from build123d import *

# Parameters (mm, degrees)
SKETCH1_W           = 463.88
SKETCH1_H           = 60
BOSS_EXTRUDE1_DEPTH = 3.175
SKETCH7_R           = 2.5
CUT_EXTRUDE5_DEPTH  = 448.729854963
SKETCH2_R           = 1.25
SKETCH2_R_2         = 1.5
SKETCH2_W           = 103
SKETCH2_H           = 37
CUT_EXTRUDE1_DEPTH  = 448.729854963
SKETCH3_W           = 158.75
SKETCH3_H           = 44.7
CUT_EXTRUDE2_DEPTH  = 448.729854963
SKETCH4_R           = 18
SKETCH4_W           = 38.5
SKETCH4_H           = 30.5
CUT_EXTRUDE3_DEPTH  = 448.729854963
SKETCH5_W           = 31.25
SKETCH5_H           = 6.35
SKETCH5_W_2         = 20
SKETCH5_W_3         = 74.25
SKETCH5_W_4         = 59.87
BOSS_EXTRUDE2_DEPTH = 3.175
SKETCH6_R           = 1.5
CUT_EXTRUDE4_DEPTH  = 449.624949735
SKETCH8_R           = 1
CUT_EXTRUDE7_DEPTH  = 449.624949735
CHAMFER2_SIZE       = 0.8


with BuildPart() as part:
    # Sketch1 → Boss-Extrude1 (new body)
    with BuildSketch(Plane(origin=(0, 0, 0), x_dir=(-1, 0, 0), z_dir=(0, 0, -1))):
        with Locations((-211.74, 30)):
            Rectangle(SKETCH1_W, SKETCH1_H)
    extrude(amount=BOSS_EXTRUDE1_DEPTH)

    # Sketch7 → Cut-Extrude5 (cut, through all)
    with BuildSketch(Plane(origin=(0, 0, -3.175), x_dir=(-1, 0, 0), z_dir=(0, 0, -1))):
        with Locations((-433.68, 50)):
            Circle(SKETCH7_R)
        with Locations((-433.68, 10)):
            Circle(SKETCH7_R)
        with Locations((10.2, 10)):
            Circle(SKETCH7_R)
        with Locations((10.2, 50)):
            Circle(SKETCH7_R)
    extrude(amount=-CUT_EXTRUDE5_DEPTH, mode=Mode.SUBTRACT)

    # Sketch2 → Cut-Extrude1 (cut, through all)
    with BuildSketch(Plane(origin=(0, 0, -3.175), x_dir=(-1, 0, 0), z_dir=(0, 0, -1))):
        with Locations((-106.378679656, 39)):
            Circle(SKETCH2_R)
        with Locations((-222.5, 49)):
            Circle(SKETCH2_R_2)
        with Locations((-222.5, 29)):
            Circle(SKETCH2_R_2)
        with Locations((-166, 37.5)):
            Rectangle(SKETCH2_W, SKETCH2_H)
        with BuildLine():
            Line((-217.5, 13), (-217.5, 18.9))
            Line((-217.5, 18.9), (-214.5, 18.9))
            Line((-214.5, 18.9), (-214.5, 13))
            ThreePointArc((-214.5, 13), (-216, 11.5), (-217.5, 13))
        make_face()
    extrude(amount=-CUT_EXTRUDE1_DEPTH, mode=Mode.SUBTRACT)

    # Sketch3 → Cut-Extrude2 (cut, through all)
    with BuildSketch(Plane(origin=(0, 0, -3.175), x_dir=(-1, 0, 0), z_dir=(0, 0, -1))):
        with Locations((-336.745, 26.05)):
            Rectangle(SKETCH3_W, SKETCH3_H)
    extrude(amount=-CUT_EXTRUDE2_DEPTH, mode=Mode.SUBTRACT)

    # Sketch4 → Cut-Extrude3 (cut, through all)
    with BuildSketch(Plane(origin=(0, 0, -3.175), x_dir=(-1, 0, 0), z_dir=(0, 0, -1))):
        with Locations((-60.25, 20.25)):
            Circle(SKETCH4_R)
        with BuildLine():
            Line((-77.75, 4.25), (-77.75, 5.25))
            ThreePointArc((-77.75, 5.25), (-76.25, 6.75), (-74.75, 5.25))
            Line((-74.75, 5.25), (-74.75, 4.25))
            ThreePointArc((-74.75, 4.25), (-76.25, 2.75), (-77.75, 4.25))
        make_face()
        with BuildLine():
            Line((-77.75, 36.25), (-77.75, 37.25))
            ThreePointArc((-77.75, 37.25), (-76.25, 38.75), (-74.75, 37.25))
            Line((-74.75, 37.25), (-74.75, 36.25))
            ThreePointArc((-74.75, 36.25), (-76.25, 34.75), (-77.75, 36.25))
        make_face()
        with BuildLine():
            Line((-16.7, 3.5), (-16.7, 4.5))
            ThreePointArc((-16.7, 4.5), (-15.2, 6), (-13.7, 4.5))
            Line((-13.7, 4.5), (-13.7, 3.5))
            ThreePointArc((-13.7, 3.5), (-15.2, 2), (-16.7, 3.5))
        make_face()
        with BuildLine():
            Line((-5.9, 4.5), (-5.9, 5.5))
            ThreePointArc((-5.9, 5.5), (-4.4, 7), (-2.9, 5.5))
            Line((-2.9, 5.5), (-2.9, 4.5))
            ThreePointArc((-2.9, 4.5), (-4.4, 3), (-5.9, 4.5))
        make_face()
        with Locations((-20.75, 23.75)):
            Rectangle(SKETCH4_W, SKETCH4_H)
    extrude(amount=-CUT_EXTRUDE3_DEPTH, mode=Mode.SUBTRACT)

    # Sketch5 → Boss-Extrude2 (add)
    with BuildSketch(Plane(origin=(0, 0, -3.175), x_dir=(-1, 0, 0), z_dir=(0, 0, -1))):
        with Locations((-65.875, -3.175)):
            Rectangle(SKETCH5_W, SKETCH5_H)
        with Locations((-9.8, -3.175)):
            Rectangle(SKETCH5_W_2, SKETCH5_H)
        with Locations((-87.375, 63.175)):
            Rectangle(SKETCH5_W_3, SKETCH5_H)
        with Locations((-237.435, 63.175)):
            Rectangle(SKETCH5_W_4, SKETCH5_H)
        with Locations((-237.435, -3.175)):
            Rectangle(SKETCH5_W_4, SKETCH5_H)
        with Locations((-413.68, 63.175)):
            Rectangle(SKETCH5_W_2, SKETCH5_H)
        with Locations((-413.68, -3.175)):
            Rectangle(SKETCH5_W_2, SKETCH5_H)
    extrude(amount=-BOSS_EXTRUDE2_DEPTH)

    # Sketch6 → Cut-Extrude4 (cut, through all)
    with BuildSketch(Plane(origin=(0, 0, -3.175), x_dir=(-1, 0, 0), z_dir=(0, 0, -1))):
        with Locations((-247.37, 50)):
            Circle(SKETCH6_R)
        with Locations((-233.5, 10)):
            Circle(SKETCH6_R)
    extrude(amount=-CUT_EXTRUDE4_DEPTH, mode=Mode.SUBTRACT)

    # Sketch8 → Cut-Extrude7 (cut, through all)
    with BuildSketch(Plane(origin=(0, 0, -3.175), x_dir=(-1, 0, 0), z_dir=(0, 0, -1))):
        with Locations((-415.412893219, 47.692893219)):
            Circle(SKETCH8_R)
        with Locations((-258.077106781, 47.692893219)):
            Circle(SKETCH8_R)
        with Locations((-258.077106781, 4.407106781)):
            Circle(SKETCH8_R)
        with Locations((-415.412893219, 4.407106781)):
            Circle(SKETCH8_R)
        with Locations((-216.792893219, 55.292893219)):
            Circle(SKETCH8_R)
        with Locations((-115.207106781, 55.292893219)):
            Circle(SKETCH8_R)
        with Locations((-115.207106781, 19.707106781)):
            Circle(SKETCH8_R)
        with Locations((-424.387106781, 60.707106781)):
            Circle(SKETCH8_R)
        with Locations((-402.972893219, 60.707106781)):
            Circle(SKETCH8_R)
        with Locations((-268.077106781, 60.707106781)):
            Circle(SKETCH8_R)
        with Locations((-206.792893219, 60.707106781)):
            Circle(SKETCH8_R)
        with Locations((-125.207106781, 60.707106781)):
            Circle(SKETCH8_R)
        with Locations((-49.542893219, 60.707106781)):
            Circle(SKETCH8_R)
        with Locations((0.907106781, -0.707106781)):
            Circle(SKETCH8_R)
        with Locations((-20.507106781, -0.707106781)):
            Circle(SKETCH8_R)
        with Locations((-49.542893219, -0.707106781)):
            Circle(SKETCH8_R)
        with Locations((-82.207106781, -0.707106781)):
            Circle(SKETCH8_R)
        with Locations((-206.792893219, -0.707106781)):
            Circle(SKETCH8_R)
        with Locations((-268.077106781, -0.707106781)):
            Circle(SKETCH8_R)
        with Locations((-402.972893219, -0.707106781)):
            Circle(SKETCH8_R)
        with Locations((-424.387106781, -0.707106781)):
            Circle(SKETCH8_R)
        with Locations((-39.292893219, 38.292893219)):
            Circle(SKETCH8_R)
        with Locations((-2.207106781, 38.292893219)):
            Circle(SKETCH8_R)
        with Locations((-39.292893219, 9.207106781)):
            Circle(SKETCH8_R)
        with Locations((-2.207106781, 9.207106781)):
            Circle(SKETCH8_R)
    extrude(amount=-CUT_EXTRUDE7_DEPTH, mode=Mode.SUBTRACT)

    # Chamfer2
    chamfer2_edges = [part.edges().sort_by_distance(p)[0] for p in [
        (81.5, -6.35, -1.5875),
        (50.25, -6.35, -1.5875),
        (19.8, -6.35, -1.5875),
        (-0.2, -6.35, -1.5875),
        (124.5, 66.35, -1.5875),
        (50.25, 66.35, -1.5875),
        (267.37, 66.35, -1.5875),
        (207.5, 66.35, -1.5875),
        (267.37, -6.35, -1.5875),
        (207.5, -6.35, -1.5875),
        (423.68, -6.35, -1.5875),
        (403.68, -6.35, -1.5875),
        (403.68, 66.35, -1.5875),
        (423.68, 66.35, -1.5875),
    ]]
    chamfer(chamfer2_edges, length=CHAMFER2_SIZE)


solid = part.part
The listing builds one solid part. Answer for the finished solid, in the listing's coordinates (mm). Give positions to 0.01 mm unless a question says otherwise; leave off trailing zeros. Loops run counter-clockwise (first coordinate to the right, second up) from the corner with the lowest first, then second, coordinate; pieces in that order, holes last.
Item 1: Each of these flat-tipped pins is pushed along its axis until it touches: pin 1 Ø1 at (y, z) = (63, -2) entering from -X; pin 2 Ø2 at (x, y) = (106.38, 39) entering from +Z; pin 3 Ø1 at (x, z) = (430.5, -2.5) entering from -Y. Where does it stop, or does it pass through?
Derived:
pin 1: stops at x = 50.25
pin 2: passes through
pin 3: stops at y = 0
Item 2: A cutting plane is placed at A-A (x = 293.5). Give the vertices of the cut face in (y, z) (3 decimals), then the cut area to 3 significant figures.
Derived:
outline: (0, -3.175) - (3.7, -3.175) - (3.7, 0) - (0, 0) - close; (48.4, -3.175) - (60, -3.175) - (60, 0) - (48.4, 0) - close
area: 48.6 mm2
Item 3: Find the intervals of material crossed by line 1 along X through (y, z) = (-3, -0.7); line 2 along Y through (x, z) = (20, -2.9); line 3 along Y through (x, z) = (368.5, -0.4), in increasing order.
Derived:
line 1: x = -0.2 to 19.8, 50.25 to 81.5, 207.5 to 267.37, 403.68 to 423.68
line 2: y = 0.15 to 8.5, 39 to 60
line 3: y = 0 to 3.7, 48.4 to 60
Item 4: A cutting plane is placed at B-B (z = -1.35). Give the number of separate pieces and of enclosed holes in the cut face, then the cut area to 3 significant figures.
Derived:
separate pieces: 1
enclosed holes: 18
area: 16,400 mm2
Item 5: Determine the mould class of faces 1 (the flat face through (215, 6, 0)), 2 (the cylindrical face through (74.534, 9.297, -1.61)) for opening direction Y: +Y half, -Y half, draft (parallel to the pull), parting line (faces both ways), or undercut.
Derived:
face 1: draft
face 2: undercut
